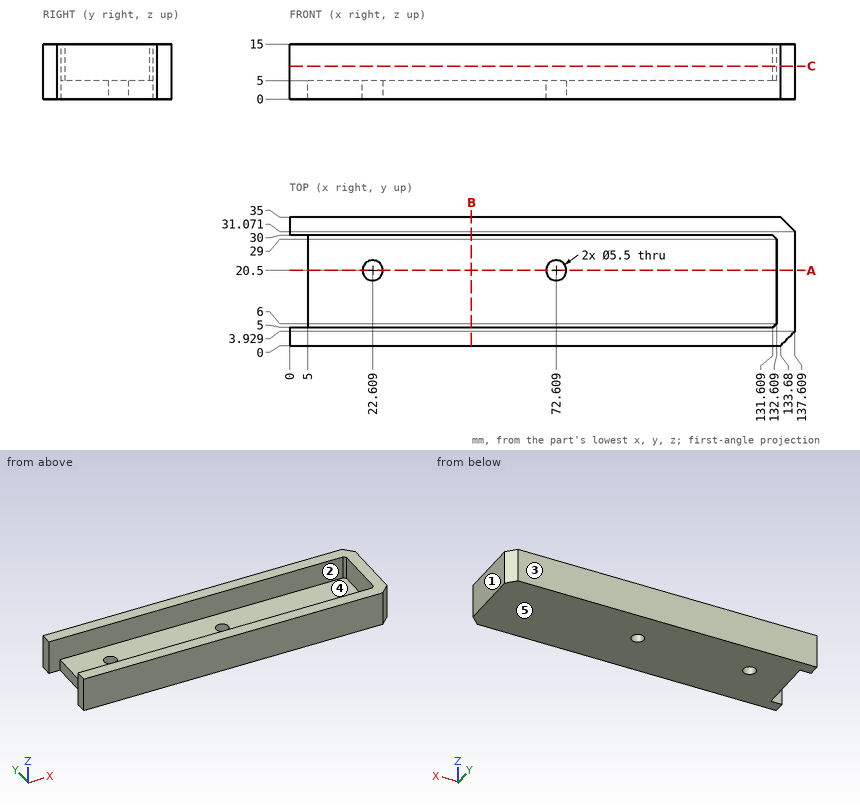
Study the drawing (mm; zero at the part's minimum x, y, z) and answer. A direction names the side the tool comes from. Coordinates: 2 decimals unless noted, no trailing zeros. Order: outer loops, then holes, each group sorted by start corner. A loop starts at its lowest first (then second) coordinate and runs counter-clockwise, first axis right, second up. Notation, with made-up numbers: M 75.5,-13 L 115.5,-13 A7 cw 115.5,-5 Z; hole C 49.5,10 d10. An arc over 180 degrees is marked long. Use CSV: the item, a comma, the result in double quotes.
Q1. Section C-C (z = 9) is taken. Determine the outline of the cut face in (x, y).
Here are the results:
outline,"M 0,0 L 133.68,0 L 137.61,3.93 L 137.61,31.07 L 133.68,35 L 0,35 L 0,30 L 131.61,30 L 132.61,29 L 132.61,6 L 131.61,5 L 0,5 Z"
Q2. Section B-B (x = 49.5) is taken. Determine the outline of the cut face in (y, z), then the cut area to 3 significant figures.
Here are the results:
outline,"M 0,0 L 35,0 L 35,15 L 30,15 L 30,5 L 5,5 L 5,15 L 0,15 Z"
area,"275 mm2"
Q3. Section A-A (y = 20.5) is taken. Determine the outline of the cut face in (x, z), then the cut area to 3 significant figures.
Here are the results:
outline,"M 5,0 L 19.86,0 L 19.86,5 L 5,5 Z; M 25.36,0 L 69.86,0 L 69.86,5 L 25.36,5 Z; M 75.36,0 L 137.61,0 L 137.61,15 L 132.61,15 L 132.61,5 L 75.36,5 Z"
area,"658 mm2"
Q4. Determine the mould class of the marked faces 1, 2 and 3 for opening direction Y: pulls with the +Y half, pulls with the -Y half, needs draft (parallel to the pull), parting line crosses it, or undercut.
Here are the results:
face 1,"needs draft"
face 2,"undercut"
face 3,"pulls with the +Y half"
Q5. Straight lines are drawn through the part: L1, parallel to X at y = 20.5, z = 2.85; L2, parallel to Y at x = 9, z = 10.75; L3, parallel to X at y = 18, z = 1 (1 decimal). For each, find the intervals that lie inside material, in ascending order.
Here are the results:
L1,"5 to 19.86, 25.36 to 69.86, 75.36 to 137.61"
L2,"0 to 5, 30 to 35"
L3,"5 to 21.5, 23.8 to 71.5, 73.8 to 137.6"
Q6. Given pin 1 Ø8 at (y, z) = (12.5, 3) entering from -X; pin 2 Ø5 at (y, z) = (14.5, 11.5) entering from -X; pin 3 Ø1 at (x, y) = (51, 21.5) entering from +Z, each flat-ended and moving along its own axis, determine where each tip first touches the part or whether it passes through.
Here are the results:
pin 1,"x = 5"
pin 2,"x = 132.61"
pin 3,"z = 5"
Q7. A tool of negligible diameter and unlimited length cuts with its end or side. For the marked faces 4 and 5, from which of +Z, -Z, +X, -X, +Y, -Y can it reach the whole face along a straight path? Write none if from no direction.
Here are the results:
face 4,"+Z, -X"
face 5,"-Z, +X, -X, +Y, -Y"
